CAD build for the part. Positions are in the model's coordinates, mm. A direction names the side the tool comes from. Give positions to 0.01 mm unless a question says otherwise; leave off trailing zeros. Loops run counter-clockwise (first coordinate to the right, second up) from the corner with the lowest first, then second, coordinate; pieces in that order, holes last.
Autodesk Inventor part; units mm, degrees
ref_plane "YZ Plane" through (0, 0, 0) normal (1, 0, 0) x (0, 1, 0)
ref_plane "XZ Plane" through (0, 0, 0) normal (0, 1, 0) x (-1, 0, 0)
ref_plane "XY Plane" through (0, 0, 0) normal (0, 0, 1) x (1, 0, 0)
sketch "スケッチ1" plane through (0, 0, 0) normal (1, 0, 0) x (0, 1, 0)
  line L0 (0, 0) -> (15, 0)
  line L1 (15, 0) -> (15, -15)
  line L2 (15, -15) -> (0, -15)
  line L3 (0, -15) -> (0, 0)
  line L4 (0, 18) -> (-5, 18)
  line L5 (-5, 18) -> (-5, -33)
  line L6 (-5, -33) -> (0, -33)
  line L7 (0, -33) -> (0, 18)
  line L8 (12, 3.5) -> (34, 3.5)
  line L9 (34, 3.5) -> (34, -18.5)
  line L10 (34, -18.5) -> (12, -18.5)
  line L11 (12, -18.5) -> (12, 3.5)
  circle A0 centre (15.5, 0) radius 1.25
  line L12 (23, 3.5) -> (23, -18.5)
  line L13 (34, -7.5) -> (12, -7.5)
  circle A1 centre (15.5, -15) radius 1.25
  circle A2 centre (30.5, 0) radius 1.25
  circle A3 centre (30.5, -15) radius 1.25
  circle A4 centre (23, -7.5) radius 6.25
  line L14 (0, 18) -> (34, 3.5)
  line L15 (34, -18.5) -> (0, -33)
  line L16 (0, 18) -> (5, 18)
  line L17 (5, 18) -> (34, 3.5)
  line L18 (0, -33) -> (5, -33)
  line L19 (5, -33) -> (34, -18.5)
  dimension "d0" = 15
  dimension "d1" = 15
  dimension "d2" = 5
  dimension "d3" = 51
  dimension "d4" = 18
  dimension "d5" = 0
  dimension "d6" = 22
  dimension "d7" = 22
  dimension "d8" = 3.5
  dimension "d9" = 3
  dimension "d10" = 2.5
  dimension "d11" = 3.5
  dimension "d12" = 3.5
  dimension "d13" = 12.5
  dimension "d18" = 5
extrude "押し出し1" add sketch "スケッチ1" against normal blind 5 contours L7 L14 L8 L11 L0 | L0 L11 L2 L3 | L11 L8 L12 A4 L13 L1 A0 L0 | L0 A0 L1 L13 L11 | L2 L11 L10 L15 L7 | L16 L17 L14 | L13 L1 A1 L2 L11 | L2 A1 L1 L13 A4 L12 L10 L11 | L15 L19 L18 | L9 L13 A4 L12 L8 | L10 L12 A4 L13 L9
fillet "フィレット2" radius 2 6 edges at (-2.5, 0, -33) (-2.5, 5, -33) (-2.5, 34, -18.5) (-2.5, 34, 3.5) (-2.5, 0, 18) (-2.5, 5, 18)
sketch "スケッチ3" plane through (0, 0, -31) normal (0, -1, 0) x (1, 0, 0)
  line L0 (0, 29.75) -> (0, 17.25)
  line L1 (0, 23.5) -> (-5, 23.5)
  line L2 (-5, 17.25) -> (-5, 29.75)
  line L3 (0, 47) -> (0, 0)
  line L4 (0, 33.5) -> (-5, 33.5)
  line L5 (0, 13.5) -> (-5, 13.5)
  point P0 (0, 31)
  point P1 (-2.5, 33.5)
  point P2 (-2.5, 23.5)
  point P3 (-2.5, 13.5)
  dimension "d20" = 10
  dimension "d21" = 2.5
  dimension "d22" = 2.5
hole "穴1" at (-2.5, 0, 2.5) at (-2.5, 0, -7.5) at (-2.5, 0, -17.5) direction (0, 1, 0) diameter 2.5 depth 5 tip angle 118
properties part number "belt_liner_v2_Plate_21" material "アルミニウム 6061"
1. Pull direction Z, two halves, no side cores. Call faces 1 (the face through (-2.46, 18.04, -11.3)), 2 (the face through (-2.54, 33.71, -18.3)), 3 (the face through (-2, 19, 11)), 4 (the face through (-5, 13, -7)): released by +Z, released by -Z, zero draft, split by the parting line, or undercut.
Responses:
face 1: undercut
face 2: released by -Z
face 3: released by +Z
face 4: zero draft
2. Tool access for faces 5 (the face through (-2.54, 33.69, 3.33)), 6 (the face through (-2.88, 2.54, 1.31)): list every direction of +Z, -Z, +X, -X, +Y, -Y with a clear straight run to the whole face (end or side of a thin tool).
Responses:
face 5: +Z, +X, -X, +Y
face 6: -Y
3. Saw through at B-B, the plane z = -15. List the corners of the cut face in (x, y), and give its area (3 significant figures).
Responses:
outline: (-5, 0) - (0, 0) - (0, 14.25) - (-5, 14.25) - close; (-5, 16.75) - (0, 16.75) - (0, 29.25) - (-5, 29.25) - close; (-5, 31.75) - (0, 31.75) - (0, 34) - (-5, 34) - close
area: 145 mm2
4. Saw through at C-C, the plane y = 23. List the corners of the cut face in (x, z), and give its area (4 significant figures).
Responses:
outline: (-5, -24) - (0, -24) - (0, -13.75) - (-5, -13.75) - close; (-5, -1.25) - (0, -1.25) - (0, 9) - (-5, 9) - close
area: 102.5 mm2
5. Saw through at D-D, the plane y = 3.5. List the corners of the cut face in (x, z), and give its area (3 significant figures).
Responses:
outline: (-5, -33) - (0, -33) - (0, 18) - (-5, 18) - close; hole circle Ø2.5 at (-2.5, -17.5); hole circle Ø2.5 at (-2.5, -7.5); hole circle Ø2.5 at (-2.5, 2.5)
area: 240 mm2
6. Drop flat-ended pins along their axis: pin 1 (2 mm diameter, centred on x = -2.5, z = -7.5, fed in from -Y); pin 2 (1.5 mm diameter, centred on x = -2.5, y = 18.5, fed in from +Z) (3 decimals); pin 3 (2 mm diameter, centred on x = -3, y = 28.5, fed in from -Z). Give the stop position or say it passes through.
Responses:
pin 1: stops at y = 5.15
pin 2: stops at z = 11.625
pin 3: stops at z = -21.75
7. Saw through at A-A, the plane y = 15.5. List the corners of the cut face in (x, z).
Responses:
outline: (-5, -27.75) - (0, -27.75) - (0, -16.25) - (-5, -16.25) - close; (-5, -13.75) - (0, -13.75) - (0, -1.25) - (-5, -1.25) - close; (-5, 1.25) - (0, 1.25) - (0, 12.75) - (-5, 12.75) - close
8. Probe line 1 along Z through (x, y) = (-2.5, 2.4); line 2 along Z through (x, y) = (-3.65, 16); line 3 along Y through (x, z) = (-2.05, -1). List the from-to ranges inside material, lowest first.
Responses:
line 1: z = -33 to -18.75, -16.25 to -8.75, -6.25 to 1.25, 3.75 to 18
line 2: z = -27.5 to -16.15, -13.85 to -1.15, 1.15 to 12.5
line 3: y = 0 to 14.75, 16.25 to 29.75, 31.25 to 34
